```python
from build123d import *

# Parameters (mm, degrees)
CROQUIS2_R            = 2.25
CORTAR_EXTRUIR1_DEPTH = 21.75
REDONDEO1_R           = 3
REDONDEO2_R           = 10


with BuildPart() as part:
    # Croquis1 → Revolución4 (revolve)
    with BuildSketch(Plane(origin=(0, 0, 0), x_dir=(0, 0, -1), z_dir=(1, 0, 0))):
        Polygon((15.75, 38), (-15.75, 38), (-15.75, 26), (-10.75, 26), (-5, 6), (-5, 0), (5, 0), (5, 6), (10.75, 26), (15.75, 26), align=None)
    revolve(axis=Axis((0, 0, -5), (0, 0, 1)))

    # Croquis2 → Cortar-Extruir1 (cut, through all)
    with BuildSketch(Plane(origin=(0, 0, -5), x_dir=(-1, 0, 0), z_dir=(0, 0, -1))):
        Circle(CROQUIS2_R)
    extrude(amount=-CORTAR_EXTRUIR1_DEPTH, mode=Mode.SUBTRACT)

    # Redondeo1
    redondeo1_edges = [part.edges().sort_by_distance(p)[0] for p in [
        (0, -38, 15.75),
        (0, -26, 15.75),
        (0, -26, -15.75),
        (0, -38, -15.75),
    ]]
    fillet(redondeo1_edges, radius=REDONDEO1_R)

    # Redondeo2
    redondeo2_edges = [part.edges().sort_by_distance(p)[0] for p in [
        (0, -6, 5),
        (0, -6, -5),
    ]]
    fillet(redondeo2_edges, radius=REDONDEO2_R)


solid = part.part
```
Could you check a few things on this model? Use its own coordinates, in mm. A direction names the side the tool comes from. Give positions to 0.01 mm unless a question says otherwise; leave off trailing zeros. Loops run counter-clockwise (first coordinate to the right, second up) from the corner with the lowest first, then second, coordinate; pieces in that order, holes last. Notation, with made-up numbers: (1, 5) - (42, 5) arc R23 cw to (42, 37) - close; hole circle Ø10 at (-8.75, 79.5). An arc over 180 degrees is marked (long way). Answer in a Markdown table with one row per item. Add a question column.
Q1. If we section it at A-A (z = -3): List the corners of the cut face in (x, y) for me, plus the area to 3 significant figures.
Q2. Which directions (+Z, -Z, +X, -X, +Y, -Y) give clear straight access to the entire face, cutting with the end or side of a thin tool? Please do faces 5 (the face through (-26.1, -13.1, 15.75)), 6 (the face through (15.821, -20.633, 11.736)).
Q3. We'd pull the mould along Y, two halves only. Please class faces 1 (the face through (0.29, 2.23, -0.07)), 2 (the face through (33.713, 17.535, 0.178)), 3 (the face through (-26.1, 13.1, -15.75)), 4 (the face through (15.821, -20.633, -11.764)): +Y half, -Y half, draft (parallel to the pull), parting line (faces both ways), or undercut.
Q4. If we section it at B-B (z = 7.5): List the corners of the cut face in (x, y) for me.
Q5. For pin 1 (12 mm diameter, centred on x = -16.5, z = 0, fed in from +Y); pin 2 (3 mm diameter, centred on y = -4.5, z = 2, fed in from +X); pin 3 (2.5 mm diameter, centred on x = 0, y = 0, fed in from -Z); pin 4 (3 mm diameter, centred on x = -29.5, z = 0.5, fed in from -Y), each with a flat end and sliding along its axis, tell me the tip position at first contact or that it passes through.
Q6. Please list where these lines run through material, in increasing order: L1, parallel to Y at x = 0, z = -11.75; L2, parallel to Y at x = 0, z = 1. Write a range as from..to.
The answers:
| question | item | result |
|---|---|---|
| 1 | outline | circle Ø76 at (0, 0); hole circle Ø4.5 at (0, 0) |
| 1 | area | 4,520 mm^2 |
| 2 | face 5 | +Z, +X, -X, +Y, -Y |
| 2 | face 6 | +Z |
| 3 | face 1 | undercut |
| 3 | face 2 | parting line |
| 3 | face 3 | draft |
| 3 | face 4 | undercut |
| 4 | outline | circle Ø76 at (0, 0); hole circle Ø29.39 at (0, 0) |
| 5 | pin 1 | stops at y = 36.52 |
| 5 | pin 2 | stops at x = 37.88 |
| 5 | pin 3 | passes through |
| 5 | pin 4 | stops at y = -25.69 |
| 6 | L1 | y = -38..-26, 26..38 |
| 6 | L2 | y = -38..-2.25, 2.25..38 |
